from build123d import *

# Parameters (mm, degrees)
SKETCH1_R           = 45
SKETCH1_R_2         = 30
SKETCH1_R_3         = 1.75
BOSS_EXTRUDE1_DEPTH = 6
SKETCH2_R           = 35.5
CUT_EXTRUDE1_DEPTH  = 3
SKETCH3_R           = 3.25
CUT_EXTRUDE2_DEPTH  = 3
CUT_EXTRUDE4_DEPTH  = 10


with BuildPart() as part:
    # Sketch1 → Boss-Extrude1 (new body)
    with BuildSketch(Plane(origin=(0, 0, 0), x_dir=(1, 0, 0), z_dir=(0, 1, 0))):
        with Locations(Location((0, 0, 0), (0, 0, 270))):
            Circle(SKETCH1_R)
        with Locations(Location((0, 0, 0), (0, 0, 270))):
            Circle(SKETCH1_R_2, mode=Mode.SUBTRACT)
        with Locations(Location((0, 40, 0), (0, 0, 270))):
            Circle(SKETCH1_R_3, mode=Mode.SUBTRACT)
        with Locations(Location((20, 34.641016151, 0), (0, 0, 270))):
            Circle(SKETCH1_R_3, mode=Mode.SUBTRACT)
        with Locations(Location((34.641016151, 20, 0), (0, 0, 270))):
            Circle(SKETCH1_R_3, mode=Mode.SUBTRACT)
        with Locations(Location((40, 0, 0), (0, 0, 270))):
            Circle(SKETCH1_R_3, mode=Mode.SUBTRACT)
        with Locations(Location((34.641016151, -20, 0), (0, 0, 270))):
            Circle(SKETCH1_R_3, mode=Mode.SUBTRACT)
        with Locations(Location((20, -34.641016151, 0), (0, 0, 270))):
            Circle(SKETCH1_R_3, mode=Mode.SUBTRACT)
        with Locations(Location((0, -40, 0), (0, 0, 270))):
            Circle(SKETCH1_R_3, mode=Mode.SUBTRACT)
        with Locations(Location((-20, -34.641016151, 0), (0, 0, 270))):
            Circle(SKETCH1_R_3, mode=Mode.SUBTRACT)
        with Locations(Location((-34.641016151, -20, 0), (0, 0, 270))):
            Circle(SKETCH1_R_3, mode=Mode.SUBTRACT)
        with Locations(Location((-40, 0, 0), (0, 0, 270))):
            Circle(SKETCH1_R_3, mode=Mode.SUBTRACT)
        with Locations(Location((-34.641016151, 20, 0), (0, 0, 270))):
            Circle(SKETCH1_R_3, mode=Mode.SUBTRACT)
        with Locations(Location((-20, 34.641016151, 0), (0, 0, 270))):
            Circle(SKETCH1_R_3, mode=Mode.SUBTRACT)
    extrude(amount=BOSS_EXTRUDE1_DEPTH)

    # Sketch2 → Cut-Extrude1 (cut)
    with BuildSketch(Plane.XZ):
        with Locations(Location((0, 0, 0), (0, 0, 270))):
            Circle(SKETCH2_R)
    extrude(amount=-CUT_EXTRUDE1_DEPTH, mode=Mode.SUBTRACT)

    # Sketch3 → Cut-Extrude2 (cut)
    with BuildSketch(Plane(origin=(0, 6, 0), x_dir=(1, 0, 0), z_dir=(0, 1, 0))):
        with Locations(Location((40, 0, 0), (0, 0, 270))):
            Circle(SKETCH3_R)
        with Locations(Location((34.641016151, -20, 0), (0, 0, 270))):
            Circle(SKETCH3_R)
        with Locations(Location((20, -34.641016151, 0), (0, 0, 270))):
            Circle(SKETCH3_R)
        with Locations(Location((0, -40, 0), (0, 0, 270))):
            Circle(SKETCH3_R)
        with Locations(Location((-20, -34.641016151, 0), (0, 0, 270))):
            Circle(SKETCH3_R)
        with Locations(Location((-34.641016151, -20, 0), (0, 0, 270))):
            Circle(SKETCH3_R)
        with Locations(Location((-40, 0, 0), (0, 0, 270))):
            Circle(SKETCH3_R)
        with Locations(Location((-34.641016151, 20, 0), (0, 0, 270))):
            Circle(SKETCH3_R)
        with Locations(Location((-20, 34.641016151, 0), (0, 0, 270))):
            Circle(SKETCH3_R)
        with Locations(Location((0, 40, 0), (0, 0, 270))):
            Circle(SKETCH3_R)
        with Locations(Location((20, 34.641016151, 0), (0, 0, 270))):
            Circle(SKETCH3_R)
        with Locations(Location((34.641016151, 20, 0), (0, 0, 270))):
            Circle(SKETCH3_R)
    extrude(amount=-CUT_EXTRUDE2_DEPTH, mode=Mode.SUBTRACT)

    # Sketch5 → Cut-Extrude4 (cut)
    with BuildSketch(Plane(origin=(0, 0, 0), x_dir=(1, 0, 0), z_dir=(0, 1, 0))):
        with BuildLine():
            Line((38.890872965, 38.890872965), (0, 0))
            Line((0, 0), (-38.890872965, 38.890872965))
            ThreePointArc((-38.890872965, 38.890872965), (0, 55), (38.890872965, 38.890872965))
        make_face()
    extrude(amount=CUT_EXTRUDE4_DEPTH, mode=Mode.SUBTRACT)


solid = part.part
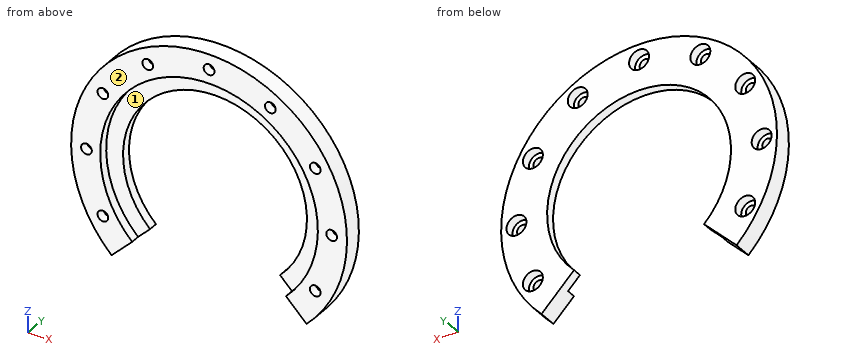
Input: part model. Units: mm. Frame: model coordinates. Face numbers are marked on the shaded views. Coordinates: 2 decimals unless noted, no trailing zeros. Loops run counter-clockwise (first coordinate to the right, second up) from the corner with the lowest first, then second, coordinate; pieces in that order, holes last.
(1) Section C-C on y = 1.5. Count the separate pieces of the cut face and the enclosed holes in it, then the cut area to 3 significant figures.
(2) First-contact query: pin 1 Ø5 at (x, z) = (34.64, 20) entering from +Y; pin 2 Ø1 at (x, y) = (-27, 1.5) entering from +Z; pin 3 Ø2 at (x, z) = (27.5, 17) entering from -Y. Flat tips, straight axial feed; report the tip coordinate or a pass-through.
(3) Section B-B on z = 0. Return the cut outline in (x, y).
(4) Pull-direction query (Z, two-part tool) for the marked faces 1 and 2; classes: released by +Z, released by -Z, zero draft, split by the parting line, or undercut.
(5) Section A-A on x = 0. Return the cut outline in (y, z), then the cut area to 3 significant figures.
(6) Section D-D on z = 8. Return the cut outline in (x, y).
(7) Material intervals for probe 1 along X at (y, z) = (1.75, 20); probe 2 along Z at (x, y) = (35, 3.5); probe 3 along Z at (x, y) = (22, 4), sorted ascending.
Data:
1. separate pieces: 1
1. enclosed holes: 9
1. area: 1,720 mm2
2. pin 1: stops at y = 3
2. pin 2: stops at z = 36.37
2. pin 3: stops at y = 3
3. outline: (-45, 0) - (-41.75, 0) - (-41.75, 3) - (-43.25, 3) - (-43.25, 6) - (-45, 6) - close; (-38.25, 0) - (-35.5, 0) - (-35.5, 3) - (-30, 3) - (-30, 6) - (-36.75, 6) - (-36.75, 3) - (-38.25, 3) - close; (30, 3) - (35.5, 3) - (35.5, 0) - (38.25, 0) - (38.25, 3) - (36.75, 3) - (36.75, 6) - (30, 6) - close; (41.75, 0) - (45, 0) - (45, 6) - (43.25, 6) - (43.25, 3) - (41.75, 3) - close
4. face 1: undercut
4. face 2: zero draft
5. outline: (0, 35.5) - (3, 35.5) - (3, 30) - (6, 30) - (6, 36.75) - (3, 36.75) - (3, 38.25) - (0, 38.25) - close; (0, 41.75) - (3, 41.75) - (3, 43.25) - (6, 43.25) - (6, 45) - (0, 45) - close
5. area: 43.5 mm2
6. outline: (-44.28, 0) - (-34.59, 0) - (-34.59, 3) - (-28.91, 3) - (-28.91, 6) - (-44.28, 6) - close; (28.91, 3) - (34.59, 3) - (34.59, 0) - (44.28, 0) - (44.28, 6) - (28.91, 6) - close
7. probe 1: x = -40.31 to -36.39, -32.89 to -29.33, 29.33 to 32.89, 36.39 to 40.31
7. probe 2: z = -28.28 to -23.23, -16.77 to 16.77, 23.23 to 28.28
7. probe 3: z = -22 to -20.4, 20.4 to 32.08, 37.2 to 39.26
